```python
from build123d import *

# Parameters (mm, degrees)
SKETCH1_R           = 1.95
BOSS_EXTRUDE1_DEPTH = 3
BOSS_EXTRUDE2_START = 2
BOSS_EXTRUDE2_DEPTH = 2
BOSS_EXTRUDE3_DEPTH = 1


with BuildPart() as part:
    # Sketch1 → Boss-Extrude1 (new body)
    with BuildSketch(Plane(origin=(0, 0, 0), x_dir=(1, 0, 0), z_dir=(0, 1, 0))):
        with BuildLine():
            Line((-49, 6), (49, 6))
            ThreePointArc((49, 6), (55, 0), (49, -6))
            Line((49, -6), (-49, -6))
            ThreePointArc((-49, -6), (-55, 0), (-49, 6))
        make_face()
        with Locations(Location((-51.5, 0, 0), (0, 0, 270))):
            Circle(SKETCH1_R, mode=Mode.SUBTRACT)
        with Locations(Location((51.5, 0, 0), (0, 0, 270))):
            Circle(SKETCH1_R, mode=Mode.SUBTRACT)
    extrude(amount=BOSS_EXTRUDE1_DEPTH)

    # Sketch2 → Boss-Extrude2 (add)
    with BuildSketch(Plane.XZ.offset(BOSS_EXTRUDE2_START)):
        with BuildLine():
            Line((54.920031913, -0.976330963), (53.491858429, -3.45))
            Line((53.491858429, -3.45), (49.508141571, -3.45))
            Line((49.508141571, -3.45), (47.516283143, 0))
            Line((47.516283143, 0), (49.508141571, 3.45))
            Line((49.508141571, 3.45), (53.491858429, 3.45))
            Line((53.491858429, 3.45), (54.920031913, 0.976330963))
            ThreePointArc((54.920031913, 0.976330963), (52.882139502, 4.574821624), (49, 6))
            Line((49, 6), (47, 6))
            Line((47, 6), (47, -6))
            Line((47, -6), (49, -6))
            ThreePointArc((49, -6), (52.882139502, -4.574821624), (54.920031913, -0.976330963))
        make_face()
        with BuildLine():
            Line((-49, -6), (-47, -6))
            Line((-47, -6), (-47, 6))
            Line((-47, 6), (-49, 6))
            ThreePointArc((-49, 6), (-52.882139502, 4.574821624), (-54.920031913, 0.976330963))
            Line((-54.920031913, 0.976330963), (-53.491858429, 3.45))
            Line((-53.491858429, 3.45), (-49.508141571, 3.45))
            Line((-49.508141571, 3.45), (-47.516283143, 0))
            Line((-47.516283143, 0), (-49.508141571, -3.45))
            Line((-49.508141571, -3.45), (-53.491858429, -3.45))
            Line((-53.491858429, -3.45), (-54.920031913, -0.976330963))
            ThreePointArc((-54.920031913, -0.976330963), (-52.882139502, -4.574821624), (-49, -6))
        make_face()
    extrude(amount=-BOSS_EXTRUDE2_DEPTH)

    # Sketch3 → Boss-Extrude3 (add)
    with BuildSketch(Plane(origin=(0, 3, 0), x_dir=(1, 0, 0), z_dir=(0, 1, 0))):
        Polygon((-32.930804426, 6), (-43, -6), (-38, -6), (-27.930804426, 6), align=None)
        Polygon((-17.930804426, 6), (-22.930804426, 6), (-33, -6), (-28, -6), align=None)
        Polygon((-7.930804426, 6), (-12.930804426, 6), (-23, -6), (-18, -6), align=None)
        Polygon((2.069195574, 6), (-2.930804426, 6), (-13, -6), (-8, -6), align=None)
        Polygon((12.069195574, 6), (7.069195574, 6), (-3, -6), (2, -6), align=None)
        Polygon((22.069195574, 6), (17.069195574, 6), (7, -6), (12, -6), align=None)
        Polygon((32.069195574, 6), (27.069195574, 6), (17, -6), (22, -6), align=None)
        Polygon((37.069195574, 6), (27, -6), (32, -6), (37.034597787, 0), align=None)
    extrude(amount=BOSS_EXTRUDE3_DEPTH)


solid = part.part
```
Model file for the job. Use its own axes, mm. A direction names the side the tool comes from. Coordinates: 2 decimals unless noted, no trailing zeros. Loops run counter-clockwise (first coordinate to the right, second up) from the corner with the lowest first, then second, coordinate; pieces in that order, holes last. Notation, with made-up numbers: (-23, 80) - (15, 80) arc R19 cw to (15, 115) - close; hole circle Ø5 at (36, -36). An arc over 180 degrees is marked (long way). Answer as a JSON object with one key per item and string values. Group by question number.
(1) Cut at B-B (x = 51.5). Give the cut face in (y, z), then the cut area to 3 significant figures.
(2) Flat gauge pins, fed straight in: pin 1 (0.6 mm diameter, centred on x = 50.5, y = -1, fed in from -Z); pin 2 (3.5 mm diameter, centred on x = 51.5, z = 0, fed in from +Y); pin 3 (0.6 mm diameter, centred on y = -1, z = -3, fed in from -X); pin 4 (1 mm diameter, centred on y = -0.5, z = 2.5, fed in from +X). Where does each tip first touch, or does it go through?
(3) Probe line 1 along X through (y, z) = (1.25, 0); line 2 along Y through (x, z) = (26.5, 0.75); line 3 along Y through (x, z) = (-11, -4). List the from-to ranges inside material, lowest first.
(4) Cut at C-C (x = 18). Give the cut face in (y, z).
(5) Tool access for faces 1 (the face through (53.144, 1.479, 1.048)), 2 (the face through (22.105, 3.493, -0.084)), 3 (the face through (-48.5, -1, -1.7)): list every direction of +Z, -Z, +X, -X, +Y, -Y with a clear straight run to the whole face (end or side of a thin tool).
(6) Two-plate mould, pull along Z, no slides. Class faces 4 (the face through (34, 4, 1)), 5 (the face through (30, 3, 0)), 6 (the face through (-33.036, 3.493, 0.084)): released by +Z, released by -Z, zero draft, split by the parting line, or undercut.
(7) Cut at A-A (y = 1.8). Give the cut face in (x, z).
(8) Cut at D-D (x = -40.5). Give the cut face in (y, z), then the cut area to 3 significant figures.
Geometry says:
{
 "1": {"outline": "(-2, -5.45) - (3, -5.45) - (3, -1.95) - (0, -1.95) - (0, -3.45) - (-2, -3.45) - close; (-2, 3.45) - (0, 3.45) - (0, 1.95) - (3, 1.95) - (3, 5.45) - (-2, 5.45) - close", "area": "29.0 mm^2"},
 "2": {"pin 1": "stops at z = -5.88", "pin 2": "passes through", "pin 3": "stops at x = -54.36", "pin 4": "stops at x = 54.66"},
 "3": {"line 1": "x = -55 to -53.45, -49.55 to 49.55, 53.45 to 55", "line 2": "y = 0 to 3", "line 3": "y = 0 to 4"},
 "4": {"outline": "(0, -6) - (4, -6) - (4, -1.15) - (3, -1.15) - (3, 4.81) - (4, 4.81) - (4, 6) - (0, 6) - close"},
 "5": {"face 1": "+Y, -Y", "face 2": "+Y", "face 3": "-Y"},
 "6": {"face 4": "zero draft", "face 5": "undercut", "face 6": "undercut"},
 "7": {"outline": "(-49, -6) - (49, -6) arc R6 ccw to (49, 6) - (-49, 6) arc R6 ccw to start; hole circle Ø3.9 at (-51.5, 0); hole circle Ø3.9 at (51.5, 0)"},
 "8": {"outline": "(0, -6) - (3, -6) - (3, 3.02) - (4, 3.02) - (4, 6) - (0, 6) - close", "area": "39.0 mm^2"}
}
